The listing builds one solid part. Answer for the finished solid, in the listing's coordinates (mm). A direction names the side the tool comes from. Round coordinates to 2 decimals unless told otherwise and drop trailing zeros. Write each loop counter-clockwise with the first axis right and the second up, starting at its lowest first coordinate (ties: lowest second). Pieces come first, ordered by that corner, then holes. Notation, with made-up numbers: (15.25, 1) - (19.25, 1) arc R19 cw to (19.25, 35) - close; hole circle Ø8 at (-35.75, 38.25). An arc over 180 degrees is marked (long way). Return JSON: item names as keys, results as strings. Group by question number.
from build123d import *

# Parameters (mm, degrees)
F1_DEPTH  = 12.7
F2_W      = 19.05
F2_H      = 88.9
F3_DEPTH  = 109.573695
F4_W      = 38.1
F4_H      = 12.7
F5_DEPTH  = 203.201
F6_W      = 12.7
F6_H      = 38.1
F7_DEPTH  = 80.187348
F8_W      = 15.60564
F8_H      = 38.1
F9_DEPTH  = 80.187348
F11_DEPTH = 25.401
F12_W     = 16.686348
F12_H     = 12.7
F13_DEPTH = 152.401
F14_W     = 16.686348
F14_H     = 12.7
F15_DEPTH = 152.401


with BuildPart() as f1:
    # F0 (on Front) → F1 (new body, symmetric)
    with BuildSketch(Plane.XZ):
        Polygon((25.4, 101.6), (0, 101.6), (-25.4, 101.6), (-25.4, 50.8), (-54.786348, 50.8), (-54.786348, -50.8), (-25.4, -50.8), (-25.4, -101.6), (0, -101.6), (25.4, -101.6), (25.4, -50.8), (54.786348, -50.8), (54.786348, 50.8), (25.4, 50.8), align=None)
    extrude(amount=F1_DEPTH, both=True)

    # F2 (on face) → F3 (cut, through all)
    with BuildSketch(Plane.YZ.offset(54.786348)):
        Rectangle(F2_W, F2_H)
    extrude(amount=-F3_DEPTH, mode=Mode.SUBTRACT)

    # F4 (on face) → F5 (cut, through all)
    with BuildSketch(Plane(origin=(0, 0, -101.6), x_dir=(1, 0, 0), z_dir=(0, 0, -1))):
        Rectangle(F4_W, F4_H)
    extrude(amount=-F5_DEPTH, mode=Mode.SUBTRACT)

    # F6 (on face) → F7 (cut, through all)
    with BuildSketch(Plane.YZ.offset(25.4)):
        with Locations((0, 76.2)):
            Rectangle(F6_W, F6_H)
    extrude(amount=-F7_DEPTH, mode=Mode.SUBTRACT)

    # F8 (on face) → F9 (cut, through all)
    with BuildSketch(Plane(origin=(-25.4, 0, 0), x_dir=(0, -1, 0), z_dir=(-1, 0, 0))):
        with Locations((0, -76.2)):
            Rectangle(F8_W, F8_H)
    extrude(amount=-F9_DEPTH, mode=Mode.SUBTRACT)

    # F10 (on face) → F11 (cut, through all)
    with BuildSketch(Plane.XZ.offset(12.7)):
        Polygon((19.05, 95.25), (-19.05, 95.25), (-19.05, 44.45), (-48.436348, 44.45), (-48.436348, -44.45), (-19.05, -44.45), (-19.05, -95.25), (19.05, -95.25), (19.05, -44.45), (48.436348, -44.45), (48.436348, 44.45), (19.05, 44.45), align=None)
    extrude(amount=-F11_DEPTH, mode=Mode.SUBTRACT)

    # F12 (on face) → F13 (cut, through all)
    with BuildSketch(Plane.XY.offset(50.8)):
        with Locations((-40.093174, 0)):
            Rectangle(F12_W, F12_H)
    extrude(amount=-F13_DEPTH, mode=Mode.SUBTRACT)

    # F14 (on face) → F15 (cut, through all)
    with BuildSketch(Plane.XY.offset(50.8)):
        with Locations((40.093174, 0)):
            Rectangle(F14_W, F14_H)
    extrude(amount=-F15_DEPTH, mode=Mode.SUBTRACT)


solid = f1.part
(1) Find section A-A (x = -44.5). Write down the section's boundary in (y, z).
(2) Consider line 1 (X direction, y = 5, z = -49.5); line 2 (Z direction, x = -8.5, y = 10.25); line 3 (X direction, y = -7.75, z = 49). Determine where each line is inside the solid, lowest interval first.
(3) Determine the mould class of faces 4 (the flat face through (19.05, 8, -65)), 5 (the flat face through (0, -6.35, 98)) for opening direction Y: +Y half, -Y half, draft (parallel to the pull), parting line (faces both ways), or undercut.
(4) Flat-ended cylindrical pins translate along their axes: pin 1 (8 mm diameter, centred on x = 35, y = -4.5, fed in from -Z); pin 2 (8 mm diameter, centred on y = -5, z = -70, fed in from +X); pin 3 (8 mm diameter, centred on y = -0.5, z = 76.5, fed in from +X). Find the tip coordinate at first contact, or state that the pin passes through.
(5) Find section D-D (z = 54). Write down the section's boundary in (x, y), plus the area to 3 significant figures.
(6) Find section B-B (z = -34.5). Write down the section's boundary in (x, y) (3 decimals).
(7) Find section C-C (x = 29.5). Write down the section's boundary in (y, z).
(8) For faces 1 (the flat face through (-22, 0, -57.15)), 2 (the flat face through (40, 6.35, 48)), 3 (the flat face through (-19.05, -9, -64)), determine the directions among +Z, -Z, +X, -X, +Y, -Y from which every point of the face is accessible in a straight line to the end or side of a thin tool.
Check sheet entries:
{
 "1": {"outline": "(-12.7, -50.8) - (-6.35, -50.8) - (-6.35, -44.45) - (-12.7, -44.45) - close; (-12.7, 44.45) - (-6.35, 44.45) - (-6.35, 50.8) - (-12.7, 50.8) - close; (6.35, -50.8) - (12.7, -50.8) - (12.7, -44.45) - (6.35, -44.45) - close; (6.35, 44.45) - (12.7, 44.45) - (12.7, 50.8) - (6.35, 50.8) - close"},
 "2": {"line 1": "x = -54.79 to -48.44, -31.75 to -19.05, 19.05 to 31.75, 48.44 to 54.79", "line 2": "z = -101.6 to -95.25, 95.25 to 101.6", "line 3": "x = -54.79 to -19.05, 19.05 to 54.79"},
 "3": {"face 4": "draft", "face 5": "undercut"},
 "4": {"pin 1": "stops at z = -50.8", "pin 2": "stops at x = 25.4", "pin 3": "passes through"},
 "5": {"outline": "(-25.4, -12.7) - (-19.05, -12.7) - (-19.05, 12.7) - (-25.4, 12.7) - close; (19.05, -12.7) - (25.4, -12.7) - (25.4, 12.7) - (19.05, 12.7) - close", "area": "323 mm^2"},
 "6": {"outline": "(-54.786, -12.7) - (-48.436, -12.7) - (-48.436, -9.525) - (-54.786, -9.525) - close; (-54.786, 9.525) - (-48.436, 9.525) - (-48.436, 12.7) - (-54.786, 12.7) - close; (48.436, -12.7) - (54.786, -12.7) - (54.786, -9.525) - (48.436, -9.525) - close; (48.436, 9.525) - (54.786, 9.525) - (54.786, 12.7) - (48.436, 12.7) - close"},
 "7": {"outline": "(-12.7, -50.8) - (12.7, -50.8) - (12.7, -44.45) - (-12.7, -44.45) - close; (-12.7, 44.45) - (12.7, 44.45) - (12.7, 50.8) - (-12.7, 50.8) - close"},
 "8": {"face 1": "+X, -X", "face 2": "+Z, -Z", "face 3": "+Y, -Y"}
}
